Design review of the part built by this model. Coordinates are the model's own, in mm. Face numbers are marked on the shaded views. Coordinates: 2 decimals unless noted, no trailing zeros. Write each loop counter-clockwise with the first axis right and the second up, starting at its lowest first coordinate (ties: lowest second). Pieces come first, ordered by that corner, then holes. Notation, with made-up numbers: (-38.75, 66) - (-6.75, 66) arc R27 ccw to (-6.75, 92) - close; hole circle Ø7 at (-3.5, 40). An arc over 180 degrees is marked (long way). Use a Markdown table: item, result.
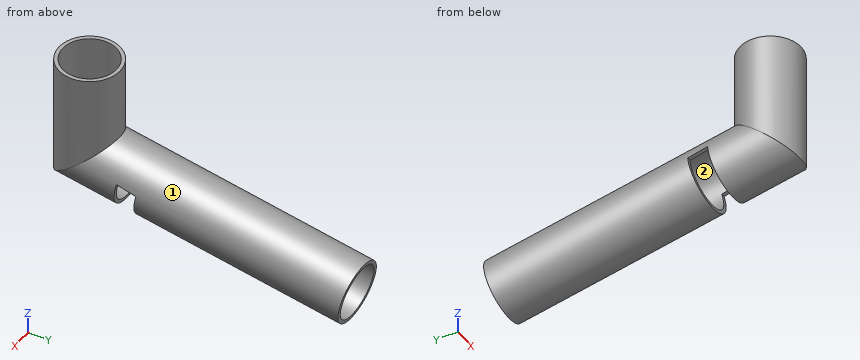
from build123d import *

# Parameters (mm, degrees)
SKETCH3_R               = 25
SKETCH3_R_2             = 22
CUT_EXTRUDE2_DEPTH      = 26
CUT_EXTRUDE2_DEPTH_BACK = 26


with BuildPart() as part:
    # Sweep1: sweep along a path in Sketch1
    with BuildLine(Plane(origin=(0, 0, 0), x_dir=(0, 0, -1), z_dir=(1, 0, 0))) as sweep1_path:
        Line((0, 0), (80, 0))
        Line((80, 0), (118.202599087, 216.657705663))
    # Sketch3 → Sweep1 (sweep)
    with BuildSketch(Plane.XY):
        Circle(SKETCH3_R)
        Circle(SKETCH3_R_2, mode=Mode.SUBTRACT)
    sweep(path=sweep1_path.line, transition=Transition.RIGHT)

    # Sketch4 → Cut-Extrude2 (cut, two sides)
    with BuildSketch(Plane(origin=(0, 0, 0), x_dir=(0, 0, -1), z_dir=(1, 0, 0))) as cut_extrude2_sk:
        Polygon((110.842308967, 30.946164041), (113.687194162, 47.080309724), (94.794337041, 50.411630176), (84.524899127, 52.222409157), (80.652201417, 36.269494553), align=None)
    extrude(amount=CUT_EXTRUDE2_DEPTH, mode=Mode.SUBTRACT)
    extrude(cut_extrude2_sk.sketch, amount=-CUT_EXTRUDE2_DEPTH_BACK, mode=Mode.SUBTRACT)


solid = part.part
(1) Take a section at C-C on x = 0. Write out the cut boundary in (y, z), and give its area (3 significant figures).
Determined:
| item | result |
|---|---|
| outline | (-25, -100.98) - (30.95, -110.84) - (31.47, -107.89) - (-22, -98.46) - (-22, 0) - (-25, 0) - close; (22, -61.54) - (220.48, -96.54) - (221, -93.58) - (25, -59.02) - (25, 0) - (22, 0) - close; (47.08, -113.69) - (212.32, -142.82) - (212.84, -139.87) - (47.6, -110.73) - close |
| area | 1,750 mm2 |
(2) Take a section at B-B on z = -41. Write out the cut boundary in (x, y).
Determined:
| item | result |
|---|---|
| outline | circle Ø50 at (0, 0); hole circle Ø44 at (0, 0) |
(3) Draft analysis for pull direction Y (two halves, no side actions). For the marked faces 1 and 2, state which applies: +Y half, -Y half, draft (parallel to the pull), parting line (faces both ways), or undercut.
Determined:
| item | result |
|---|---|
| face 1 | parting line |
| face 2 | undercut |
(4) Take a section at A-A on x = -15.5. Write out the cut boundary in (y, z).
Determined:
| item | result |
|---|---|
| outline | (-19.62, -96.46) - (31.88, -105.54) - (32.58, -101.6) - (-15.61, -93.1) - (-15.61, 0) - (-19.62, 0) - close; (15.61, -66.9) - (219.37, -102.83) - (220.06, -98.89) - (19.62, -63.54) - (19.62, 0) - (15.61, 0) - close; (48.02, -108.38) - (213.25, -137.52) - (213.95, -133.58) - (48.71, -104.44) - close |
(5) For pin 1 (8 mm diameter, centred on x = 7.5, z = -64.5, fed in from -Y); pin 2 (10 mm diameter, centred on x = -4.5, y = 5, fed in from -Z); pin 3 (12 mm diameter, centred on x = 6.5, z = -36.5, fed in from -Y) (3 decimals), all flat-tipped, find the tip position at first contact; note any pin that passes through.
Determined:
| item | result |
|---|---|
| pin 1 | y = -24.75 |
| pin 2 | z = -106.95 |
| pin 3 | y = -24.995 |
(6) For L1, parallel to Y at x = 0, z = -55; L2, parallel to X at y = 191, z = -102, list the stretches that pass through material, from the lowest coordinate up. Write a range as from..to.
Determined:
| item | result |
|---|---|
| L1 | -25..-22, 22..25 |
| L2 | -22.2..-18.75, 18.75..22.2 |
